Design review of the part built by this model. Coordinates are the model's own, in mm. Face numbers are marked on the shaded views. A direction names the side the tool comes from. Give positions to 0.01 mm unless a question says otherwise; leave off trailing zeros. Loops run counter-clockwise (first coordinate to the right, second up) from the corner with the lowest first, then second, coordinate; pieces in that order, holes last. Notation, with made-up numbers: (70, 22) - (95, 22) arc R17 ccw to (95, 41) - close; hole circle Ø4 at (66.5, -12.75). An arc over 180 degrees is marked (long way). Put each result on its own line as item: value. Start each with the question number.
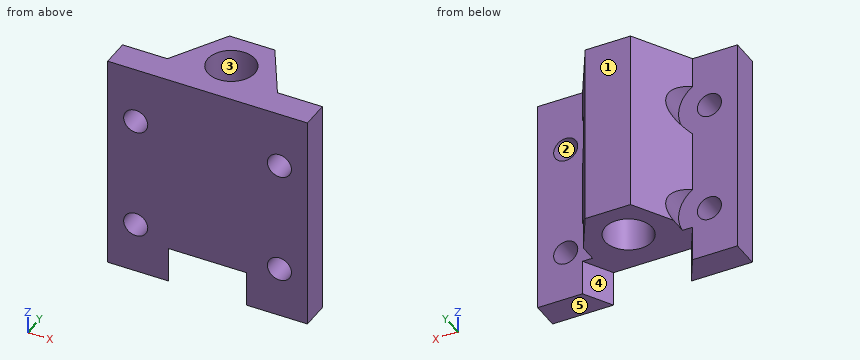
Autodesk Inventor part; units mm, degrees
ref_plane "Work Plane3" through (-75.5066, 299.1132, 245.5159) normal (0, 0, 1) x (1, 0, 0)
ref_plane "YZ Plane" through (0, 0, 0) normal (1, 0, 0) x (0, 1, 0)
ref_plane "XZ Plane" through (0, 0, 0) normal (0, 1, 0) x (-1, 0, 0)
ref_plane "Work Plane2" through (234.4934, -62.0868, 206.5159) normal (0, 0, -1) x (-1, 0, 0)
sketch "Sketch3" plane through (234.4934, -62.0868, 206.5159) normal (0, 0, -1) x (-1, 0, 0)
  circle A0 centre (324.3, 410) radius 4 construction
  line L0 (314.485, 407) -> (320.2585, 417)
  line L1 (320.2585, 417) -> (328.3415, 417)
  line L2 (328.3415, 417) -> (334.115, 407)
  line L3 (-385, 402) -> (385, 402) construction
  line L4 (314.485, 407) -> (314.485, 402) construction
  line L5 (334.115, 407) -> (334.115, 402) construction
  line L6 (314.485, 407) -> (306.485, 407)
  line L7 (306.485, 407) -> (306.485, 402)
  line L8 (306.485, 402) -> (314.485, 402)
  line L9 (314.485, 402) -> (314.485, 407) construction
  line L10 (334.115, 407) -> (342.115, 407)
  line L11 (342.115, 407) -> (342.115, 402)
  line L12 (342.115, 402) -> (334.115, 402)
  line L13 (334.115, 402) -> (334.115, 407) construction
  line L14 (314.485, 402) -> (334.115, 402)
  point P0 (234.4934, 62.0868)
  dimension "d19" = 8
  dimension "d20" = 3
  dimension "d21" = 60
  dimension "d22" = 60
  dimension "d24" = 3
  dimension "d25" = 3
  dimension "d26" = 5
  dimension "d27" = 5
  dimension "d28" = 8
  dimension "d29" = 8
ref_plane "Work Plane3" through (-75.5066, 299.1132, 245.5159) normal (0, 0, 1) x (1, 0, 0)
extrude "Extrusion2" add sketch "Sketch3" against normal up to surface (39 mm away)
sketch "Sketch4" plane through (234.4934, -62.0868, 206.5159) normal (0, 0, -1) x (-1, 0, 0)
  point P0 (234.4934, 62.0868)
  point P1 (324.3, 410)
hole "Hole2" at (-89.8066, 347.9132, 206.5159) direction (0, 0, 1) diameter 8.4 end through all counterbore diameter 18 counterbore depth 6.3
sketch "Sketch5" plane through (-79.9916, 344.9132, 206.5159) normal (0, 1, 0) x (1, 0, 0)
  line L0 (-119.515, -29) -> (748.485, -29) construction
  line L1 (-119.515, -9) -> (748.485, -9) construction
  line L2 (8, 0) -> (8, -39) construction
  line L3 (-27.6299, 0) -> (-27.6299, -39) construction
  point P0 (79.9916, 206.5159)
  point P1 (3, -29)
  point P2 (-22.6299, -29)
  point P3 (-22.6299, -9)
  point P4 (3, -9)
  dimension "d39" = 5
  dimension "d40" = 5
  dimension "d41" = 5
  dimension "d42" = 5
hole "Hole3" at (-76.9916, 344.9132, 235.5159) at (-102.6215, 344.9132, 235.5159) at (-102.6215, 344.9132, 215.5159) at (-76.9916, 344.9132, 215.5159) direction (0, -1, 0) diameter 4.3 end through all
sketch "Sketch6" plane through (-79.9916, 344.9132, 206.5159) normal (0, 1, 0) x (1, 0, 0)
  point P0 (79.9916, 206.5159)
  point P1 (3, -29)
  point P2 (-22.6299, -29)
  point P3 (-22.6299, -9)
  point P4 (3, -9)
hole "Hole4" at (-76.9916, 344.9132, 235.5159) at (-102.6215, 344.9132, 235.5159) at (-102.6215, 344.9132, 215.5159) at (-76.9916, 344.9132, 215.5159) direction (0, 1, 0) diameter 11 end through all
sketch "Sketch7" plane through (234.4934, -62.0868, 206.5159) normal (0, 0, -1) x (-1, 0, 0)
  arc A0 (315.4094, 408.601) -> (320.1769, 402) centre (324.3, 410) ccw
  line L0 (315.4094, 408.601) -> (314.485, 407)
  line L1 (314.485, 407) -> (306.485, 407)
  line L2 (306.485, 407) -> (306.485, 402)
  line L3 (306.485, 402) -> (320.1769, 402)
  arc A1 (328.4231, 402) -> (333.1906, 408.601) centre (324.3, 410) ccw
  line L4 (328.4231, 402) -> (342.115, 402)
  line L5 (342.115, 402) -> (342.115, 407)
  line L6 (342.115, 407) -> (334.115, 407)
  line L7 (334.115, 407) -> (333.1906, 408.601)
  line L8 (320.2585, 417) -> (314.485, 407)
  line L9 (314.485, 407) -> (317.3718, 402)
  line L10 (306.485, 402) -> (342.115, 402)
  line L11 (342.115, 407) -> (334.115, 407)
  line L12 (334.115, 407) -> (331.2282, 402)
  point P0 (234.4934, 62.0868)
  point P1 (308.4231, 367)
  dimension "d63" = 60
  dimension "d64" = 60
extrude "Extrusion3" cut sketch "Sketch7" against normal up to surface (6.3 mm away) contours A0 L3 L9 L0 | A1 L7 L12 L4
equation "\"d22\" = d21"
equation "\"d24\" = d20"
equation "\"d25\" = d24"
equation "\"d27\" = d26"
equation "\"d29\" = d28"
properties part number "AxleHolder"
Item 1: Machinability: for the marked faces 4 and 5, which of the approach directions +Z, -Z, +X, -X, +Y, -Y give a long, thin tool a straight path to every point of the face, cutting with its end or side? Answer none if there is none.
Item 2: Consider section D-D (z = 215). State the section outline as (x, y) points.
Item 3: Consider section A-A (z = 210). State the section outline as (x, y) points, plus the area to 3 significant figures.
Item 4: For L1, parallel to Z at x = -75.5, y = 341; L2, parallel to X at y = 343, z = 216; L3, parallel to Z at x = -93, y = 342, list the stretches that pass through material, from the lowest coordinate up. Write a range as from..to.
Item 5: Consider section C-C (y = 345.5). State the section outline as (x, z) points, plus the area to 3 significant figures.
Item 6: For P1, Ø4, axis at x = -102.62, z = 215.52, coming from the -Y side; P2, Ø1, axis at y = 349, z = 216.5, coming from the +X side; P3, Ø5, axis at x = -102.62, z = 235.52, coming from the +Y side; P4, Ø2, axis at y = 346, z = 232.5, coming from the +X side, all flat-tipped, find the tip position at first contact; note any pin that passes through.
Item 7: Consider section B-B (x = -78). State the section outline as (y, z) points, plus the area to 3 significant figures.
Item 8: Mouldability with a two-part tool opening along Y and no side actions: class the marked faces 1, 2 and 3 as pulls with the +Y half, pulls with the -Y half, needs draft (parallel to the pull), parting line crosses it, or undercut.
Geometry says:
1. face 4: -Z, +Y
1. face 5: -Z, +X, -X, +Y, -Y
2. outline: (-107.62, 339.91) - (-104.71, 339.91) - (-104.71, 344.91) - (-107.62, 344.91) - close; (-100.53, 339.91) - (-79.08, 339.91) - (-79.08, 344.91) - (-82.47, 344.91) - (-82.47, 349.2) - (-85.77, 354.91) - (-93.85, 354.91) - (-97.15, 349.2) - (-97.15, 344.91) - (-100.53, 344.91) - close; (-74.9, 339.91) - (-71.99, 339.91) - (-71.99, 344.91) - (-74.9, 344.91) - close; hole circle Ø8.4 at (-89.81, 347.91)
3. outline: (-107.62, 339.91) - (-96.73, 339.91) - (-99.62, 344.91) - (-107.62, 344.91) - close; (-82.88, 339.91) - (-71.99, 339.91) - (-71.99, 344.91) - (-79.99, 344.91) - close
3. area: 94.4 mm2
4. L1: z = 206.52..213.97, 217.06..233.97, 237.06..245.52
4. L2: x = -107.62..-104.72, -100.53..-79.09, -74.9..-71.99
4. L3: z = 212.82..245.52
5. outline: (-99.28, 219.89) arc R5.5 cw to (-97.83, 212.82) - (-93.24, 212.82) - (-93.24, 245.52) - (-99.28, 245.52) - (-99.28, 239.89) arc R5.5 cw to (-99.28, 231.15) - close; (-86.37, 212.82) - (-81.78, 212.82) arc R5.5 cw to (-80.33, 219.89) - (-80.33, 231.15) arc R5.5 cw to (-80.33, 239.89) - (-80.33, 245.52) - (-86.37, 245.52) - close
5. area: 345 mm2
6. P1: passes through
6. P2: stops at x = -82.29
6. P3: stops at y = 344.91
6. P4: stops at x = -80.75
7. outline: (339.91, 206.52) - (344.91, 206.52) - (344.91, 213.62) - (339.91, 213.62) - close; (339.91, 217.41) - (344.91, 217.41) - (344.91, 233.62) - (339.91, 233.62) - close; (339.91, 237.41) - (344.91, 237.41) - (344.91, 245.52) - (339.91, 245.52) - close
7. area: 157 mm2
8. face 1: pulls with the +Y half
8. face 2: needs draft
8. face 3: undercut
